Autodesk Inventor part; units mm, degrees
ref_plane "YZ Plane" through (0, 0, 0) normal (1, 0, 0) x (0, 1, 0)
ref_plane "XZ Plane" through (0, 0, 0) normal (0, 1, 0) x (-1, 0, 0)
ref_plane "XY Plane" through (0, 0, 0) normal (0, 0, 1) x (1, 0, 0)
sketch "スケッチ1" plane through (0, 0, 0) normal (0, 0, 1) x (1, 0, 0)
  line L0 (-85, -150) -> (85, -150)
  line L1 (85, -150) -> (85, 150)
  line L2 (85, 150) -> (-85, 150)
  line L3 (-85, 150) -> (-85, -150)
  point P0 (0, 0)
  point P1 (85, 0)
  dimension "d0" = 300
  dimension "d1" = 170
  dimension "d3" = 85
  dimension "d4" = 150
extrude "押し出し1" add sketch "スケッチ1" along normal mid plane 150
sketch "スケッチ2" plane through (0, 0, -75) normal (0, 0, -1) x (-1, 0, 0)
  line L0 (85, 150) -> (85, -150)
  line L1 (85, -20) -> (65, -20)
  line L2 (65, -20) -> (65, 20)
  line L3 (65, 20) -> (85, 20)
  line L4 (85, 20) -> (85, -20)
  line L5 (-85, -150) -> (85, -150)
  point P0 (0, 0)
  dimension "d7" = 40
  dimension "d8" = 20
  dimension "d9" = 130
extrude "押し出し2" add sketch "スケッチ2" along normal blind 110
properties part number "body_luggage"
Verification items for the finished model (mm, model axes). A direction names the side the tool comes from. Give positions to 0.01 mm unless a question says otherwise; leave off trailing zeros. Order: outer loops, then holes, each group sorted by start corner. A loop starts at its lowest first (then second) coordinate and runs counter-clockwise, first axis right, second up. Notation, with made-up numbers: M 32.5,-32.5 L 45.5,-32.5 A26 cw 45.5,-9.5 Z; hole C 68.25,-38 d6. An arc over 180 degrees is marked long. Return JSON: item names as keys, results as strings. Group by question number.
1) Access from +Z, -Z, +X, -X, +Y, -Y to the whole of each face (thin tool, end or side, straight path). Record for faces 1 (the face through (-75, 20, -129)), 2 (the face through (-75, -20, -129)), 3 (the face through (-65, 0, -129)), 4 (the face through (-1, -150, -1)).
2) Section check A-A on y = -0.5. Record the cut outline in (x, z).
3) Go/stop test with flat-tipped pins: pin 1 Ø10 at (x, z) = (-74, -156.5) entering from -Y; pin 2 Ø5 at (x, y) = (27, 70) entering from -Z; pin 3 Ø16 at (x, z) = (-74.5, -112.5) entering from +Y. Record where each tip stops, or that it passes through.
4) Section check C-C on z = -148. Record the cut outline in (x, y).
5) Section check B-B on x = -58. Record the cut outline in (y, z), and give its area (3 significant figures).
6) Scan lines: line 1 (X direction, y = 13, z = -104.5); line 2 (Z direction, x = 42.5, y = -46.5); line 3 (Y direction, x = -78, z = -152). Record each from-to range of solid material in increasing order.
Answer block:
{
 "1": {"face 1": "-Z, +X, -X, +Y", "face 2": "-Z, +X, -X, -Y", "face 3": "-Z, +X, +Y, -Y", "face 4": "+Z, -Z, +X, -X, -Y"},
 "2": {"outline": "M -85,-185 L -65,-185 L -65,-75 L 85,-75 L 85,75 L -85,75 Z"},
 "3": {"pin 1": "stops at y = -20", "pin 2": "stops at z = -75", "pin 3": "stops at y = 20"},
 "4": {"outline": "M -85,-20 L -65,-20 L -65,20 L -85,20 Z"},
 "5": {"outline": "M -150,-75 L 150,-75 L 150,75 L -150,75 Z", "area": "45,000 mm^2"},
 "6": {"line 1": "x = -85 to -65", "line 2": "z = -75 to 75", "line 3": "y = -20 to 20"}
}
